```python
from build123d import *

# Parameters (mm, degrees)
F0_W     = 10
F0_H     = 10
F1_DEPTH = 33.65
F2_W     = 10
F2_H     = 10
F2_R     = 2
F3_DEPTH = 4
F4_W     = 10
F4_H     = 10
F4_R     = 2
F5_DEPTH = 4
F6_R     = 3
F7_DEPTH = 200


with BuildPart() as f1:
    # F0 (on Front) → F1 (new body, symmetric)
    with BuildSketch(Plane.XZ):
        Rectangle(F0_W, F0_H)
    extrude(amount=F1_DEPTH, both=True)

    # F2 (on face) → F3 (cut)
    with BuildSketch(Plane.XZ.offset(33.65)):
        Rectangle(F2_W, F2_H)
        Circle(F2_R, mode=Mode.SUBTRACT)
    extrude(amount=-F3_DEPTH, mode=Mode.SUBTRACT)

    # F4 (on face) → F5 (cut)
    with BuildSketch(Plane(origin=(0, 33.65, 0), x_dir=(-1, 0, 0), z_dir=(0, 1, 0))):
        Rectangle(F4_W, F4_H)
        Circle(F4_R, mode=Mode.SUBTRACT)
    extrude(amount=-F5_DEPTH, mode=Mode.SUBTRACT)

    # F6 (on face) → F7 (join)
    with BuildSketch(Plane.YZ.offset(5)):
        with BuildLine():
            ThreePointArc((0, -5), (3.535534, -3.535534), (5, 0))
            ThreePointArc((5, 0), (3.535534, 3.535534), (0, 5))
            ThreePointArc((0, 5), (-5, 0), (0, -5))
        make_face()
        Circle(F6_R, mode=Mode.SUBTRACT)
    extrude(amount=F7_DEPTH)


solid = f1.part
```
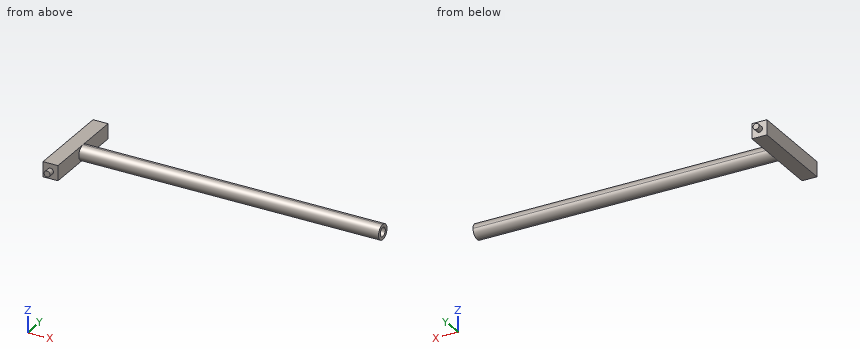
Check sheet for the modelled part. Datum: model origin and axes. Units: mm. Give positions to 0.01 mm unless a question says otherwise; leave off trailing zeros. Order: outer loops, then holes, each group sorted by start corner. A loop starts at its lowest first (then second) coordinate and runs counter-clockwise, first axis right, second up. Notation, with made-up numbers: M -3,88.5 L 47,88.5 A20 ccw 47,115.5 Z; hole C -27.5,-19.75 d2. An arc over 180 degrees is marked long. Answer in a Markdown table with one row per item. Add a question column.
Q1. Sectioned sample at B-B, the plane y = 12. Record the boundary of the cut face in (x, z).
Q2. Gauge pin test, flat ends, axial feed: pin 1 Ø5.5 at (y, z) = (0, 0) entering from +X; pin 2 Ø1.5 at (x, z) = (165, -3.5) entering from +Y; pin 3 Ø3 at (x, z) = (140.5, -1.5) entering from +Y. Record the tip position at first contact, or that the pin passes through.
Q3. Thickness scan on L1, parallel to X at y = -21, z = -1.5; L2, parallel to Y at x = 40.5, z = -4; L3, parallel to Y at x = 189.5, z = -0.75. Record the ranges inside material, lowest first.
Q4. Sectioned sample at A-A, the plane x = 0. Record the boundary of the cut face in (y, z).
Q5. Sectioned sample at C-C, the plane x = 37.5. Record the boundary of the cut face in (y, z).
Verdict:
| question | item | result |
|---|---|---|
| 1 | outline | M -5,-5 L 5,-5 L 5,5 L -5,5 Z |
| 2 | pin 1 | x = 5 |
| 2 | pin 2 | y = 4.18 |
| 2 | pin 3 | y = 5 |
| 3 | L1 | -5 to 5 |
| 3 | L2 | -3 to 3 |
| 3 | L3 | -4.94 to -2.9, 2.9 to 4.94 |
| 4 | outline | M -33.65,-2 L -29.65,-2 L -29.65,-5 L 29.65,-5 L 29.65,-2 L 33.65,-2 L 33.65,2 L 29.65,2 L 29.65,5 L -29.65,5 L -29.65,2 L -33.65,2 Z |
| 5 | outline | C 0,0 d10; hole C 0,0 d6 |
